For this review, take the finished solid that the model builds, in its own axes (mm). A direction names the side the tool comes from. Coordinates: 2 decimals unless noted, no trailing zeros. Loops run counter-clockwise (first coordinate to the right, second up) from the corner with the lowest first, then second, coordinate; pieces in that order, holes last. Notation, with made-up numbers: (-38.75, -33) -> (-34.75, -33) arc R22 cw to (-34.75, -21) -> close; hole circle Ø1 at (-36, -0.75). An arc over 180 degrees is marked (long way). One line per item, written item: value.
from build123d import *

# Parameters (mm, degrees)
F2_R     = 6.35
F3_DEPTH = 104.489224
F4_DEPTH = 76.2


with BuildPart() as f1:
    # F0 (on Front) → F1 (revolve)
    with BuildSketch(Plane.XZ):
        with BuildLine():
            Line((-3.134028, -33.796337), (-3.134028, -50.052336))
            Line((-3.134028, -50.052336), (22.265972, -50.052336))
            Line((22.265972, -50.052336), (22.265972, 29.035888))
            ThreePointArc((22.265972, 29.035888), (14.826484, 46.9964), (-3.134028, 54.435888))
            Line((-3.134028, 54.435888), (-3.134028, 38.179888))
            ThreePointArc((-3.134028, 38.179888), (3.331756, 35.501672), (6.009972, 29.035888))
            Line((6.009972, 29.035888), (6.009972, -33.796337))
            Line((6.009972, -33.796337), (-3.134028, -33.796337))
        make_face()
    revolve(axis=Axis((-3.134028, 0, 2.191776), (0, 0, -1)))

    # F2 (on face) → F3 (cut, through all)
    with BuildSketch(Plane(origin=(0, 0, -50.052336), x_dir=(1, 0, 0), z_dir=(0, 0, -1))):
        with Locations((-3.134028, 0)):
            Circle(F2_R)
    extrude(amount=-F3_DEPTH, mode=Mode.SUBTRACT)

    # F2 (on face) → F4 (join)
    with BuildSketch(Plane(origin=(0, 0, -50.052336), x_dir=(1, 0, 0), z_dir=(0, 0, -1))):
        with Locations((-3.134028, 0)):
            Circle(F2_R)
    extrude(amount=-F4_DEPTH)


solid = f1.part
1. Take a section at B-B, the plane z = 27.5. Give the boundary of the cut face in (x, y), and give its area (3 significant figures).
Return value:
outline: circle Ø50.8 at (-3.13, 0); hole circle Ø18.29 at (-3.13, 0)
area: 1,760 mm2
2. The part is to be moulded in two halves that separate along Z. For faces 4 (the flat face through (-3, 0, 26.148)), 5 (the cylindrical face through (-6.441, -25.184, -9.955)), 6 (the cylindrical face through (-0.2, 5.63, -4.24)), say which applies: pulls with the +Z half, pulls with the -Z half, needs draft (parallel to the pull), parting line crosses it, or undercut.
Return value:
face 4: pulls with the +Z half
face 5: needs draft
face 6: undercut
3. Insertion check: pin 1 Ø2 at (x, z) = (-9, 11.5) entering from -Y; pin 2 Ø2 at (y, z) = (-16, -34.5) entering from +X; pin 3 Ø6 at (y, z) = (-15, 17) entering from +X; pin 4 Ø14.5 at (x, y) = (-7, 3) entering from +Z. Each pin has a flat end and moves straight along its axis. Give the tip position at first contact, or say it passes through.
Return value:
pin 1: stops at y = -24.93
pin 2: stops at x = 17.36
pin 3: stops at x = 19.25
pin 4: stops at z = 53.63
4. To check wall thickness, follow probe 1 along Y at (x, z) = (-3.5, 18.5); probe 2 along Y at (x, z) = (-8.5, 21); probe 3 along X at (y, z) = (0, 7.5). State the ranges of each line that lie inside material, in increasing order. Write a range as from..to.
Return value:
probe 1: y = -25.4..-9.14, -6.34..6.34, 9.14..25.4
probe 2: y = -24.83..-7.4, -3.4..3.4, 7.4..24.83
probe 3: x = -28.53..-12.28, -9.48..3.22, 6.01..22.27
5. Take a section at A-A, the plane z = -4.5. Give the boundary of the cut face in (x, y), and give its area (3 significant figures).
Return value:
outline: circle Ø50.8 at (-3.13, 0); circle Ø12.7 at (-3.13, 0); hole circle Ø18.29 at (-3.13, 0)
area: 1,890 mm2
6. For faces 1 (the cylindrical face through (-0.2, 5.63, 44.5)), 2 (the flat face through (-9.4, 1.9, -33.796)), 3 (the flat face through (-3, 0, -50.052)), list the 3-axis set-ups (+Z, -Z, +X, -X, +Y, -Y) from which the entire face can be reached by the end or side of a thin tool; tool diameter is ignored.
Return value:
face 1: +Z
face 2: none
face 3: -Z, +X, -X, +Y, -Y
